from build123d import *

# Parameters (mm, degrees)
SKETCH1_R          = 6.7945
SKETCH1_R_2        = 5.5245
EXTRUDE1_DEPTH     = 0.8255
CUT_EXTRUDE1_DEPTH = 0.889
CHAMFER1_SIZE      = 0.254
CHAMFER1_SIZE2     = 0.439940905


with BuildPart() as part:
    # Sketch1 → Extrude1 (new, symmetric)
    with BuildSketch(Plane.XY):
        with Locations(Location((0, 0, 0), (0, 0, 180))):
            Circle(SKETCH1_R)
        with Locations(Location((0, 0, 0), (0, 0, 180))):
            Circle(SKETCH1_R_2, mode=Mode.SUBTRACT)
    extrude(amount=EXTRUDE1_DEPTH, both=True)

    # Sketch2 → Cut-Extrude1 (cut)
    with BuildSketch(Plane.XY.offset(0.8255)):
        with BuildLine():
            Line((-0.5969, 6.768230244), (-0.5969, 5.492159014))
            ThreePointArc((-0.5969, 5.492159014), (0, 5.5245), (0.5969, 5.492159014))
            Line((0.5969, 5.492159014), (0.5969, 6.768230244))
            ThreePointArc((0.5969, 6.768230244), (0, 6.7945), (-0.5969, 6.768230244))
        make_face()
        with BuildLine():
            Line((-0.5969, -6.768230244), (-0.5969, -5.492159014))
            ThreePointArc((-0.5969, -5.492159014), (0, -5.5245), (0.5969, -5.492159014))
            Line((0.5969, -5.492159014), (0.5969, -6.768230244))
            ThreePointArc((0.5969, -6.768230244), (0, -6.7945), (-0.5969, -6.768230244))
        make_face()
    extrude(amount=-CUT_EXTRUDE1_DEPTH, mode=Mode.SUBTRACT)

    # Chamfer1
    chamfer1_edges = [part.edges().sort_by_distance(p)[0] for p in [
        (-5.011031196, -4.588550599, 0.8255),
        (6.7945, 0, -0.8255),
        (6.7945, 0, 0.8255),
    ]]
    chamfer1_side = [part.faces().sort_by_distance(p)[0] for p in [
        (6.7945, 0, 0),
    ]]
    chamfer(chamfer1_edges, length=CHAMFER1_SIZE, length2=CHAMFER1_SIZE2, reference=chamfer1_side[0])


solid = part.part
Verification items for the finished model (mm, model axes). A direction names the side the tool comes from. Give positions to 0.01 mm unless a question says otherwise; leave off trailing zeros. Write each loop counter-clockwise with the first axis right and the second up, starting at its lowest first coordinate (ties: lowest second). Pieces come first, ordered by that corner, then holes. Notation, with made-up numbers: (14, -1.75) -> (21, -1.75) arc R22 cw to (21, 28.25) -> close; hole circle Ø7 at (13.25, 28). An arc over 180 degrees is marked (long way). Use CSV: the item, a comma, the result in double quotes.
(1) Set-up check for faces 4 (the flat face through (-0.597, 6.1, 0.4)), 5 (the conical face through (6.52, -0.14, 0.73)): record each of +Z, -Z, +X, -X, +Y, -Y from which the full face is reachable in a straight line by a thin tool's end or side.
Derived:
face 4,"+Z, +Y, -Y"
face 5,"+Z, +X"
(2) Release check for a two-part mould opening along Y. For faces 1 (the cylindrical face through (4.1, -3.7, 0)), 2 (the cylindrical face through (-6.48, -2.04, 0.01)), 3 (the flat face through (5, -3, -0.826)) record: +Y half, -Y half, draft (parallel to the pull), parting line (faces both ways), or undercut.
Derived:
face 1,"undercut"
face 2,"parting line"
face 3,"draft"
(3) Sectioned sample at B-B (y = 0). Record the cut outline in (x, z).
Derived:
outline,"(-6.79, -0.57) -> (-6.35, -0.83) -> (-5.52, -0.83) -> (-5.52, 0.83) -> (-6.35, 0.83) -> (-6.79, 0.57) -> close; (5.52, -0.83) -> (6.35, -0.83) -> (6.79, -0.57) -> (6.79, 0.57) -> (6.35, 0.83) -> (5.52, 0.83) -> close"
(4) Sectioned sample at A-A (x = 0). Record the cut outline in (y, z).
Derived:
outline,"(-6.79, -0.57) -> (-6.35, -0.83) -> (-5.52, -0.83) -> (-5.52, -0.06) -> (-6.79, -0.06) -> close; (5.52, -0.83) -> (6.35, -0.83) -> (6.79, -0.57) -> (6.79, -0.06) -> (5.52, -0.06) -> close"
(5) Go/stop test with flat-tipped pins: pin 1 (0.7 mm diameter, centred on y = 6.5, z = 0.5, fed in from +X); pin 2 (1 mm diameter, centred on x = 0, y = -6, fed in from +Z). Record where each tip stops, or that it passes through.
Derived:
pin 1,"stops at x = 2.89"
pin 2,"stops at z = -0.06"
(6) Material ranges on L1, parallel to Y at x = 0, z = -0.45; L2, parallel to Y at x = 2.75, z = -0.45; L3, parallel to X at y = 3.5, z = -0.7, recorded low to high.
Derived:
L1,"y = -6.79 to -5.52, 5.52 to 6.79"
L2,"y = -6.21 to -4.79, 4.79 to 6.21"
L3,"x = -5.56 to -4.27, 4.27 to 5.56"
